```python
from build123d import *

# Parameters (mm, degrees)
EXTRUDE_233_DEPTH     = 4
CUT_EXTRUDE_382_DEPTH = 3
EXTRUDE_469_DEPTH     = 12


with BuildPart() as part:
    # 草图3 → Extrude 233 (new body)
    with BuildSketch(Plane.XY):
        with BuildLine():
            Line((-17, -55), (17, -55))
            ThreePointArc((17, -55), (19.121320344, -54.121320344), (20, -52))
            Line((20, -52), (20, 52))
            ThreePointArc((20, 52), (19.121320344, 54.121320344), (17, 55))
            Line((17, 55), (-17, 55))
            ThreePointArc((-17, 55), (-19.121320344, 54.121320344), (-20, 52))
            Line((-20, 52), (-20, -52))
            ThreePointArc((-20, -52), (-19.121320344, -54.121320344), (-17, -55))
        make_face()
    extrude(amount=EXTRUDE_233_DEPTH)

    # 草图4 → Cut-Extrude 382 (cut)
    with BuildSketch(Plane.XY):
        with BuildLine():
            Line((-16.75, -32.25), (-13.75, -32.25))
            ThreePointArc((-13.75, -32.25), (-12.335786438, -31.664213562), (-11.75, -30.25))
            Line((-11.75, -30.25), (-11.75, -24.25))
            ThreePointArc((-11.75, -24.25), (-12.335786438, -22.835786438), (-13.75, -22.25))
            Line((-13.75, -22.25), (-16.75, -22.25))
            ThreePointArc((-16.75, -22.25), (-18.164213562, -22.835786438), (-18.75, -24.25))
            Line((-18.75, -24.25), (-18.75, -30.25))
            ThreePointArc((-18.75, -30.25), (-18.164213562, -31.664213562), (-16.75, -32.25))
        make_face()
        with BuildLine():
            Line((-16.75, -1.75), (-13.75, -1.75))
            ThreePointArc((-13.75, -1.75), (-12.335786438, -1.164213562), (-11.75, 0.25))
            Line((-11.75, 0.25), (-11.75, 6.25))
            ThreePointArc((-11.75, 6.25), (-12.335786438, 7.664213562), (-13.75, 8.25))
            Line((-13.75, 8.25), (-16.75, 8.25))
            ThreePointArc((-16.75, 8.25), (-18.164213562, 7.664213562), (-18.75, 6.25))
            Line((-18.75, 6.25), (-18.75, 0.25))
            ThreePointArc((-18.75, 0.25), (-18.164213562, -1.164213562), (-16.75, -1.75))
        make_face()
        with BuildLine():
            Line((13.75, -32.25), (16.75, -32.25))
            ThreePointArc((16.75, -32.25), (18.164213562, -31.664213562), (18.75, -30.25))
            Line((18.75, -30.25), (18.75, -24.25))
            ThreePointArc((18.75, -24.25), (18.164213562, -22.835786438), (16.75, -22.25))
            Line((16.75, -22.25), (13.75, -22.25))
            ThreePointArc((13.75, -22.25), (12.335786438, -22.835786438), (11.75, -24.25))
            Line((11.75, -24.25), (11.75, -30.25))
            ThreePointArc((11.75, -30.25), (12.335786438, -31.664213562), (13.75, -32.25))
        make_face()
        with BuildLine():
            Line((13.75, -1.75), (16.75, -1.75))
            ThreePointArc((16.75, -1.75), (18.164213562, -1.164213562), (18.75, 0.25))
            Line((18.75, 0.25), (18.75, 6.25))
            ThreePointArc((18.75, 6.25), (18.164213562, 7.664213562), (16.75, 8.25))
            Line((16.75, 8.25), (13.75, 8.25))
            ThreePointArc((13.75, 8.25), (12.335786438, 7.664213562), (11.75, 6.25))
            Line((11.75, 6.25), (11.75, 0.25))
            ThreePointArc((11.75, 0.25), (12.335786438, -1.164213562), (13.75, -1.75))
        make_face()
    extrude(amount=CUT_EXTRUDE_382_DEPTH, mode=Mode.SUBTRACT)

    # 草图5 → Extrude 469 (add)
    with BuildSketch(Plane.XY):
        with BuildLine():
            Line((-19.6, -56), (19.6, -56))
            ThreePointArc((19.6, -56), (19.882842712, -55.882842712), (20, -55.6))
            Line((20, -55.6), (20, -55.4))
            ThreePointArc((20, -55.4), (19.882842712, -55.117157288), (19.6, -55))
            Line((19.6, -55), (-19.6, -55))
            ThreePointArc((-19.6, -55), (-19.882842712, -55.117157288), (-20, -55.4))
            Line((-20, -55.4), (-20, -55.6))
            ThreePointArc((-20, -55.6), (-19.882842712, -55.882842712), (-19.6, -56))
        make_face()
    extrude(amount=EXTRUDE_469_DEPTH)


solid = part.part
```
For this review, take the finished solid that the model builds, in its own axes (mm). A direction names the side the tool comes from. Give positions to 0.01 mm unless a question says otherwise; leave off trailing zeros. Write each loop counter-clockwise with the first axis right and the second up, starting at its lowest first coordinate (ties: lowest second). Pieces come first, ordered by that corner, then holes. Notation, with made-up numbers: M 30,65.5 L 40,65.5 A34 cw 40,99.5 Z; hole C -21.75,76 d5. An arc over 180 degrees is marked long. Answer as a JSON object with one key per item and string values. Group by question number.
Item 1: For probe 1 along Y at (x, z) = (16.5, 2.75); probe 2 along Z at (x, y) = (11, 30); probe 3 along Y at (x, z) = (14, 7.5), list the stretches that pass through material, from the lowest coordinate up. Write a range as [from, to].
Item 2: Consider section A-A on y = -29. Write out the cut boundary in (x, z), plus the area to 3 significant figures.
Item 3: Tool access review of faces 1 (the flat face through (0, 1, 4)), 2 (the cylindrical face through (18.15, -31.68, 1.48)), 3 (the cylindrical face through (19.14, 54.1, 1.97)): name each direction out of +Z, -Z, +X, -X, +Y, -Y from which nothing blocks a thin tool from reaching the whole face with its end or side.
Item 4: Consider section D-D on z = 1.5. Count the separate pieces of the cut face and the enclosed holes in it, plus the area to 3 significant figures.
Item 5: Consider section B-B on z = 6.75. Write out the cut boundary in (x, y), plus the area to 3 significant figures.
Item 6: For pin 1 Ø12 at (x, y) = (-10, -19) entering from +Z; pin 2 Ø5.5 at (x, y) = (16.5, -28) entering from -Z; pin 3 Ø3.5 at (x, y) = (15.5, 5.5) entering from -Z, all flat-tipped, find the tip position at first contact; note any pin that passes through.
Item 7: Consider section C-C on x = -1. Write out the cut boundary in (y, z).
Check result:
{
 "1": {"probe 1": "y = [-56, -32.25], [-22.25, -1.75], [8.25, 55]", "probe 2": "z = [0, 4]", "probe 3": "y = [-56, -55]"},
 "2": {"outline": "M -20,0 L -18.75,0 L -18.75,3 L -11.75,3 L -11.75,0 L 11.75,0 L 11.75,3 L 18.75,3 L 18.75,0 L 20,0 L 20,4 L -20,4 Z", "area": "118 mm^2"},
 "3": {"face 1": "+Z, +X, -X, +Y", "face 2": "-Z", "face 3": "+Z, -Z, +X, +Y"},
 "4": {"separate pieces": "1", "enclosed holes": "4", "area": "4,170 mm^2"},
 "5": {"outline": "M -20,-55.6 A0.4 ccw -19.6,-56 L 19.6,-56 A0.4 ccw 20,-55.6 L 20,-55.4 A0.4 ccw 19.6,-55 L -19.6,-55 A0.4 ccw -20,-55.4 Z", "area": "39.9 mm^2"},
 "6": {"pin 1": "stops at z = 4", "pin 2": "stops at z = 0", "pin 3": "stops at z = 3"},
 "7": {"outline": "M -56,0 L 55,0 L 55,4 L -55,4 L -55,12 L -56,12 Z"}
}
